Model file for the job. Use its own axes, mm. Coordinates: 2 decimals unless noted, no trailing zeros. Order: outer loops, then holes, each group sorted by start corner. A loop starts at its lowest first (then second) coordinate and runs counter-clockwise, first axis right, second up. Notation, with made-up numbers: (17.5, 18.5) - (55.5, 18.5) arc R12 ccw to (55.5, 39.5) - close; hole circle Ø1 at (67.5, 41.25). An arc over 180 degrees is marked (long way). Put each result on its own line as item: value. Start each with the question number.
```python
from build123d import *

# Parameters (mm, degrees)
F0_W     = 76.2
F0_H     = 76.2
F0_R     = 3.175
F0_R_2   = 12.7
F1_DEPTH = 6.35


with BuildPart() as f1:
    # F0 (on Front) → F1 (new body)
    with BuildSketch(Plane.XZ):
        Rectangle(F0_W, F0_H)
        with Locations((0, -25.4)):
            Circle(F0_R, mode=Mode.SUBTRACT)
        with Locations((-25.4, 0)):
            Circle(F0_R, mode=Mode.SUBTRACT)
        Circle(F0_R_2, mode=Mode.SUBTRACT)
        with Locations((25.4, 0)):
            Circle(F0_R, mode=Mode.SUBTRACT)
        with Locations((0, 25.4)):
            Circle(F0_R, mode=Mode.SUBTRACT)
    extrude(amount=F1_DEPTH)


solid = f1.part
```
Item 1: Slice it at A-A, the plane z = 25.4. Give the cut face in (x, y) (3 decimals), plus the area to 3 significant figures.
Item 2: Pull direction Z, two halves, no side cores. Call faces 1 (the face through (-1, -3, -38.1)), 2 (the face through (-2.75, -3.13, -12.4)), 3 (the face through (-1, -3, 38.1)): pulls with the +Z half, pulls with the -Z half, needs draft (parallel to the pull), parting line crosses it, or undercut.
Item 3: Slice it at B-B, the plane x = 25.4. Give the cut face in (y, z) (3 decimals), plus the area to 3 significant figures.
Item 4: Slice it at D-D, the plane x = 0. Give the cut face in (y, z) (3 decimals).
Item 5: Wall check: line 1 along Z through (x, y) = (0, -2.25) (3 decimals); line 2 along Z through (x, y) = (-25.4, -1.25) (3 decimals); line 3 along Z through (x, y) = (-2, -1.75). Give the ranges that are in metal, low to high.
Item 6: Flat gauge pin, fed straight in: pin 1 Ø5 at (x, z) = (-25.4, 0) entering from +Y. Where does the tip first touch, or does it go through?
Item 7: Slice it at C-C, the plane y = -3.25. Give the cut face in (x, z) (3 decimals).
Here are the results:
1. outline: (-38.1, -6.35) - (-3.175, -6.35) - (-3.175, 0) - (-38.1, 0) - close; (3.175, -6.35) - (38.1, -6.35) - (38.1, 0) - (3.175, 0) - close
1. area: 444 mm^2
2. face 1: pulls with the -Z half
2. face 2: undercut
2. face 3: pulls with the +Z half
3. outline: (-6.35, -38.1) - (0, -38.1) - (0, -3.175) - (-6.35, -3.175) - close; (-6.35, 3.175) - (0, 3.175) - (0, 38.1) - (-6.35, 38.1) - close
3. area: 444 mm^2
4. outline: (-6.35, -38.1) - (0, -38.1) - (0, -28.575) - (-6.35, -28.575) - close; (-6.35, -22.225) - (0, -22.225) - (0, -12.7) - (-6.35, -12.7) - close; (-6.35, 12.7) - (0, 12.7) - (0, 22.225) - (-6.35, 22.225) - close; (-6.35, 28.575) - (0, 28.575) - (0, 38.1) - (-6.35, 38.1) - close
5. line 1: z = -38.1 to -28.575, -22.225 to -12.7, 12.7 to 22.225, 28.575 to 38.1
5. line 2: z = -38.1 to -3.175, 3.175 to 38.1
5. line 3: z = -38.1 to -27.87, -22.93 to -12.54, 12.54 to 22.93, 27.87 to 38.1
6. pin 1: passes through
7. outline: (-38.1, -38.1) - (38.1, -38.1) - (38.1, 38.1) - (-38.1, 38.1) - close; hole circle Ø6.35 at (-25.4, 0); hole circle Ø25.4 at (0, 0); hole circle Ø6.35 at (0, -25.4); hole circle Ø6.35 at (0, 25.4); hole circle Ø6.35 at (25.4, 0)
